```python
from build123d import *

# Parameters (mm, degrees)
F1_DEPTH = 3.2


with BuildPart() as f1:
    # F0 (on Top) → F1 (new body)
    with BuildSketch(Plane.XY):
        with BuildLine():
            Line((0, 1.218053), (-18.579833, 1.218053))
            Line((-18.579833, 1.218053), (-18.579833, -3.544447))
            Line((-18.579833, -3.544447), (-18.579833, -8.306947))
            Line((-18.579833, -8.306947), (0, -8.306947))
            ThreePointArc((0, -8.306947), (3.912919, -5.947395), (8.407667, -5.125409))
            Line((8.407667, -5.125409), (13.170167, -5.125409))
            Line((13.170167, -5.125409), (13.170167, -1.963484))
            Line((13.170167, -1.963484), (8.407667, -1.963484))
            ThreePointArc((8.407667, -1.963484), (3.912919, -1.141499), (0, 1.218053))
        make_face()
        with BuildLine():
            Line((17.932667, -1.963484), (13.170167, -1.963484))
            Line((13.170167, -1.963484), (13.170167, -5.125409))
            Line((13.170167, -5.125409), (17.932667, -5.125409))
            ThreePointArc((17.932667, -5.125409), (22.427415, -5.947395), (26.340334, -8.306947))
            Line((26.340334, -8.306947), (44.920167, -8.306947))
            Line((44.920167, -8.306947), (44.920167, -3.544447))
            Line((44.920167, -3.544447), (44.920167, 1.218053))
            Line((44.920167, 1.218053), (26.340334, 1.218053))
            ThreePointArc((26.340334, 1.218053), (22.427415, -1.141499), (17.932667, -1.963484))
        make_face()
    extrude(amount=F1_DEPTH)


solid = f1.part
```
Geometry: final body of the model. Coordinates: model frame, mm. A direction names the side the tool comes from. Give positions to 0.01 mm unless a question says otherwise; leave off trailing zeros. Write each loop counter-clockwise with the first axis right and the second up, starting at its lowest first coordinate (ties: lowest second). Pieces come first, ordered by that corner, then holes.
1. Section query B-B, the plane z = 1.55. Return loops of the section in (x, y), then the cut area to 3 significant figures.
2. Draft query along X for faces 4 (the cylindrical face through (3.973, -1.164, 1.578)), 5 (the flat face through (13, -3, 0)), 6 (the cylindrical face through (22.488, -1.119, 1.578)), 7 (the flat face through (-18.58, -3, 2)). Return one class per face: released by +X, released by -X, zero draft, split by the parting line, or undercut.
3. Section query C-C, the plane y = -6. Return loops of the section in (x, z), then the cut area to 3 significant figures.
4. Line query: probe 1 along Y at (x, z) = (12, 1.25); probe 2 along X at (y, z) = (1, 1.1); probe 3 along X at (y, z) = (-0.25, 2.35). Output: solid intervals per line, ascending.
5. Pin query (flat end, axial travel): P1, Ø1.6, axis at x = 14, z = 2.5, coming from the -Y side; P2, Ø1, axis at x = 14, z = 1, coming from the +Y side. Return the tip coordinate at first contact, or that it passes through.
6. Section query D-D, the plane x = 15. Return loops of the section in (y, z), then the cut area to 3 significant figures.
7. Section query A-A, the plane y = 0. Return loops of the section in (x, z), then the cut area to 3 significant figures.
8. Reachability of faces 1 (the flat face through (13, -1.963, 2)), 2 (the cylindrical face through (22.367, -5.925, 1.578)), 3 (the flat face through (44.92, -4, 2)) from +Z, -Z, +X, -X, +Y, -Y: full face, straight path, thin tool, end or side. Return the list, or none.
Computed:
1. outline: (-18.58, -8.31) - (0, -8.31) arc R12.7 cw to (8.41, -5.13) - (17.93, -5.13) arc R12.7 cw to (26.34, -8.31) - (44.92, -8.31) - (44.92, 1.22) - (26.34, 1.22) arc R12.7 cw to (17.93, -1.96) - (8.41, -1.96) arc R12.7 cw to (0, 1.22) - (-18.58, 1.22) - close
1. area: 471 mm2
2. face 4: undercut
2. face 5: zero draft
2. face 6: undercut
2. face 7: released by -X
3. outline: (-18.58, 0) - (3.78, 0) - (3.78, 3.2) - (-18.58, 3.2) - close; (22.56, 0) - (44.92, 0) - (44.92, 3.2) - (22.56, 3.2) - close
3. area: 143 mm2
4. probe 1: y = -5.13 to -1.96
4. probe 2: x = -18.58 to 0.25, 26.09 to 44.92
4. probe 3: x = -18.58 to 2.04, 24.3 to 44.92
5. P1: stops at y = -5.13
5. P2: stops at y = -1.96
6. outline: (-5.13, 0) - (-1.96, 0) - (-1.96, 3.2) - (-5.13, 3.2) - close
6. area: 10.1 mm2
7. outline: (-18.58, 0) - (1.62, 0) - (1.62, 3.2) - (-18.58, 3.2) - close; (24.72, 0) - (44.92, 0) - (44.92, 3.2) - (24.72, 3.2) - close
7. area: 129 mm2
8. face 1: +Z, -Z, +Y
8. face 2: +Z, -Z, -Y
8. face 3: +Z, -Z, +X, +Y, -Y
